Input: part model. Units: mm. Frame: model coordinates. A direction names the side the tool comes from. Round coordinates to 2 decimals unless told otherwise and drop trailing zeros. Loops run counter-clockwise (first coordinate to the right, second up) from the corner with the lowest first, then second, coordinate; pieces in that order, holes last. Notation, with made-up numbers: (30.25, -31) - (79.25, -31) arc R12 cw to (79.25, -24) - close; hole circle Ø6 at (12.25, -26.75). An arc over 180 degrees is marked (long way). Use CSV: the item, a comma, the result in double quotes. Start each with the question number.
1. Cut plane B-B (x = -20). Return loops of the section in (y, z) (3 decimals).
2. Access query for faces 4 (the flat face through (-5.556, 0, 0)), 5 (the flat face through (0, 0, -60.325)). Directions: +Z, -Z, +X, -X, +Y, -Y. A direction counts if a zero-diameter tool reaches every point of the face in a straight line with its end or side. Return the directions, or none.
3. Cut plane A-A (x = 0). Return loops of the section in (y, z) (3 decimals).
4. Cut plane C-C (z = 40). Return loops of the section in (x, y) (3 decimals), and give its area (3 significant figures).
5. Pull-direction query (X, two-part tool) for faces 1 (the flat face through (31, -12.7, 33)), 2 (the flat face through (-34.925, 0, -1)), 3 (the flat face through (0, 0, 23.587)); classes: +X half, -X half, draft (parallel to the pull), parting line (faces both ways), or undercut.
6. Pin query (flat end, axial travel): P1, Ø12, axis at x = 8, z = -34, coming from the -Y side (3 decimals). Return the tip coordinate at first contact, or that it passes through.
7. Cut plane D-D (y = -9.5). Return loops of the section in (x, z) (3 decimals), and give its area (3 significant figures).
8. Material intervals for probe 1 along Z at (x, y) = (0, 0) (3 decimals); probe 2 along X at (y, z) = (2, -9) (3 decimals); probe 3 along X at (y, z) = (-3, -17) (3 decimals), sorted ascending. Write a range as from..to.
```python
from build123d import *

# Parameters (mm, degrees)
F0_R     = 3.175
F1_DEPTH = 12.7
F0_W     = 69.85
F0_H     = 120.65
F0_R_2   = 1.5875
F0_W_2   = 3.0226
F0_H_2   = 1.0957790866
F0_H_3   = 2.4735292748
F2_DEPTH = 3.175


# Not quite as in the source:
# - a feature names something its author has since deleted; it is built from what else it names


with BuildPart() as f1:
    # F0 (on Front) → F1 (new body)
    with BuildSketch(Plane.XZ):
        with Locations((30.9913528, 33.0454)):
            Circle(F0_R)
    extrude(amount=F1_DEPTH)

    # F0 (on Front) → F2 (join, symmetric)
    with BuildSketch(Plane.XZ):
        Rectangle(F0_W, F0_H)
        with Locations((0, -33.3375)):
            Circle(F0_R_2, mode=Mode.SUBTRACT)
        Polygon((1.5113, 12.7), (5.55625, 12.7), (5.55625, -12.7), (1.5113, -12.7), (1.5113, -15.1735292748), (1.5113, -25.2650182862), (-1.5113, -25.2650182862), (-1.5113, -15.1735292748), (-1.5113, -12.7), (-5.55625, -12.7), (-5.55625, 12.7), (-1.5113, 12.7), (-1.5113, 13.7957790866), (-1.5113, 23.5874790866), (1.5113, 23.5874790866), (1.5113, 13.7957790866), align=None, mode=Mode.SUBTRACT)
        with Locations((0, 33.3375)):
            Circle(F0_R_2, mode=Mode.SUBTRACT)
        with Locations((30.9913528, 33.0454)):
            Circle(F0_R, mode=Mode.SUBTRACT)
        with Locations((0, 13.2478895433)):
            Rectangle(F0_W_2, F0_H_2)
        with Locations((30.9913528, 33.0454)):
            Circle(F0_R)
        with Locations((0, -13.9367646374)):
            Rectangle(F0_W_2, F0_H_3)
    extrude(amount=F2_DEPTH, both=True)


solid = f1.part
```
Established:
1,outline,"(-3.175, -60.325) - (3.175, -60.325) - (3.175, 60.325) - (-3.175, 60.325) - close"
2,face 4,"+Y, -Y"
2,face 5,"-Z, +X, -X, +Y, -Y"
3,outline,"(-3.175, -60.325) - (3.175, -60.325) - (3.175, -34.925) - (-3.175, -34.925) - close; (-3.175, -31.75) - (3.175, -31.75) - (3.175, -25.265) - (-3.175, -25.265) - close; (-3.175, -15.174) - (3.175, -15.174) - (3.175, -12.7) - (-3.175, -12.7) - close; (-3.175, 12.7) - (3.175, 12.7) - (3.175, 13.796) - (-3.175, 13.796) - close; (-3.175, 23.587) - (3.175, 23.587) - (3.175, 31.75) - (-3.175, 31.75) - close; (-3.175, 34.925) - (3.175, 34.925) - (3.175, 60.325) - (-3.175, 60.325) - close"
4,outline,"(-34.925, -3.175) - (34.925, -3.175) - (34.925, 3.175) - (-34.925, 3.175) - close"
4,area,"444 mm2"
5,face 1,"draft"
5,face 2,"-X half"
5,face 3,"undercut"
6,P1,"stops at y = -3.175"
7,outline,"circle Ø6.35 at (30.991, 33.045)"
7,area,"31.7 mm2"
8,probe 1,"z = -60.325..-34.925, -31.75..-25.265, -15.174..-12.7, 12.7..13.796, 23.587..31.75, 34.925..60.325"
8,probe 2,"x = -34.925..-5.556, 5.556..34.925"
8,probe 3,"x = -34.925..-1.511, 1.511..34.925"
